```python
from build123d import *

# Parameters (mm, degrees)
SKETCH1_W                    = 57.15
SKETCH1_H                    = 38.1
BASE_FLANGE1_DEPTH           = 1.5875
EDGE_FLANGE1_STRIP_W         = 7.9375
EDGE_FLANGE1_STRIP_H         = 1.5875
EDGE_FLANGE1_STRIP_CUT_DEPTH = 57.15
EDGE_FLANGE1_DEPTH           = 57.15
F_1_4_CLEARANCE_HOLE1_D      = 6.7564
F_1_4_CLEARANCE_HOLE2_D      = 6.7564
BOSS_EXTRUDE1_DEPTH          = 57.15
CUT_EXTRUDE1_DEPTH           = 79.545162168
BOSS_EXTRUDE2_DEPTH          = 3.175
BOSS_EXTRUDE3_DEPTH          = 3.175


# Sheet-metal steps are written as plain solids
with BuildPart() as part:
    # Sketch1 → Base-Flange1 (new body)
    with BuildSketch(Plane(origin=(0, 0, 0), x_dir=(1, 0, 0), z_dir=(0, 1, 0))):
        with Locations((0, -19.05)):
            Rectangle(SKETCH1_W, SKETCH1_H)
    extrude(amount=BASE_FLANGE1_DEPTH)

    # Edge-Flange1 strip (across the edge) → Edge-Flange1 strip cut (cut)
    with BuildSketch(Plane(origin=(28.575, 1.5875, 0), x_dir=(0, 0, 1), z_dir=(-1, 0, 0))):
        with Locations((-1.5875, -0.79375)):
            Rectangle(EDGE_FLANGE1_STRIP_W, EDGE_FLANGE1_STRIP_H)
    extrude(amount=EDGE_FLANGE1_STRIP_CUT_DEPTH, mode=Mode.SUBTRACT)

    # Edge-Flange1 section (across the edge) → Edge-Flange1 (add)
    with BuildSketch(Plane(origin=(28.575, 1.5875, 0), x_dir=(0, 0, 1), z_dir=(-1, 0, 0))):
        with BuildLine():
            Line((0, 0.79375), (0, 36.5125))
            Line((0, 36.5125), (1.5875, 36.5125))
            Line((1.5875, 36.5125), (1.5875, 0.79375))
            ThreePointArc((1.5875, 0.79375), (1.819983992, 0.232483992), (2.38125, 0))
            Line((2.38125, 0), (2.38125, -1.5875))
            ThreePointArc((2.38125, -1.5875), (0.697451977, -0.890048023), (0, 0.79375))
        make_face()
    extrude(amount=EDGE_FLANGE1_DEPTH)

    # 1/4 Clearance Hole1 (through all)
    with Locations(Plane(origin=(0, 1.5875, 0), x_dir=(1, 0, 0), z_dir=(0, 1, 0))):
        with Locations((-15.875, -25.4), (15.875, -25.4)):
            Hole(F_1_4_CLEARANCE_HOLE1_D / 2)

    # 1/4 Clearance Hole2 (through all)
    with Locations(Plane.XY.offset(1.5875)):
        with Locations((-15.875, 25.4), (15.875, 25.4)):
            Hole(F_1_4_CLEARANCE_HOLE2_D / 2)

    # Sketch16 → Boss-Extrude1 (add, through all)
    with BuildSketch(Plane(origin=(28.575, 0, 0), x_dir=(0, 0, -1), z_dir=(1, 0, 0))):
        with BuildLine():
            Line((0, 2.38125), (0, 0))
            Line((0, 0), (-2.38125, 0))
            ThreePointArc((-2.38125, 0), (-0.697451977, 0.697451977), (0, 2.38125))
        make_face()
    extrude(amount=-BOSS_EXTRUDE1_DEPTH)

    # Sketch18 → Cut-Extrude1 (cut, through all)
    with BuildSketch(Plane(origin=(28.575, 0, 0), x_dir=(0, 0, -1), z_dir=(1, 0, 0))):
        with BuildLine():
            Line((-2.38125, 1.5875), (-1.5875, 1.5875))
            Line((-1.5875, 1.5875), (-1.5875, 2.38125))
            ThreePointArc((-1.5875, 2.38125), (-1.819983992, 1.819983992), (-2.38125, 1.5875))
        make_face()
    extrude(amount=-CUT_EXTRUDE1_DEPTH, mode=Mode.SUBTRACT)

    # Sketch21 → Boss-Extrude2 (add)
    with BuildSketch(Plane(origin=(28.575, 0, 0), x_dir=(0, 0, -1), z_dir=(1, 0, 0))):
        Polygon((-1.5875, 1.5875), (-38.1, 1.5875), (-38.1, 0), (0, 0), (0, 38.1), (-1.5875, 38.1), align=None)
    extrude(amount=-BOSS_EXTRUDE2_DEPTH)

    # Sketch22 → Boss-Extrude3 (add)
    with BuildSketch(Plane.ZY.offset(28.575)):
        Polygon((38.1, 1.5875), (1.5875, 1.5875), (1.5875, 38.1), (0, 38.1), (0, 0), (38.1, 0), align=None)
    extrude(amount=-BOSS_EXTRUDE3_DEPTH)


solid = part.part
```
The model under review builds one solid part; all positions refer to its coordinate system, in mm. A direction names the side the tool comes from. Give positions to 0.01 mm unless a question says otherwise; leave off trailing zeros. Write each loop counter-clockwise with the first axis right and the second up, starting at its lowest first coordinate (ties: lowest second). Pieces come first, ordered by that corner, then holes. Notation, with made-up numbers: (84, 62) - (127, 62) arc R17 ccw to (127, 92) - close; hole circle Ø8 at (89.25, 87.5). An arc over 180 degrees is marked (long way). Answer in a Markdown table with one row per item. Add a question column.
1. Tool access review of faces 5 (the flat face through (0, 1.588, 20)), 6 (the flat face through (0, 1, 38.1)): name each direction out of +Z, -Z, +X, -X, +Y, -Y from which nothing blocks a thin tool from reaching the whole face with its end or side.
2. We need section C-C on x = 16.5. Write out the cut boundary in (y, z), then the cut area to 3 significant figures.
3. We need section A-A on z = 25.4. Write out the cut boundary in (x, y) (1 decimal), then the cut area to 3 significant figures.
4. We need section D-D on z = 34. Write out the cut boundary in (x, y) (1 decimal).
5. Insertion check: P1, Ø6, axis at x = -6, z = 32, coming from the +Y side; P2, Ø5.5, axis at x = -15.875, y = 25.4, coming from the +Z side; P3, Ø11, axis at x = 14, y = 11, coming from the +Z side. Each pin has a flat end and moves straight along its axis. Give the tip position at first contact, or say it passes through.
6. Wall thickness on line 1 along Z through (x, y) = (-3.5, 8): over which ranges is the line inside the solid? List them lowest first. Write a range as [from, to].
7. Draft analysis for pull direction Z (two halves, no side actions). For faces 1 (the flat face through (0, 19, 0)), 2 (the flat face through (-28.575, 11, 1)), 3 (the cylindrical face through (-17.43, 0.78, 28.4)), 4 (the cylindrical face through (14.32, 0.78, 28.4)), state which applies: +Z half, -Z half, draft (parallel to the pull), parting line (faces both ways), or undercut.
Ans:
| question | item | result |
|---|---|---|
| 1 | face 5 | +Z, +X, -X, +Y |
| 1 | face 6 | +Z, +X, -X, +Y, -Y |
| 2 | outline | (0, 0) - (22.08, 0) - (22.08, 1.59) - (1.59, 1.59) - (1.59, 22.08) - (0, 22.08) - close; (0, 28.72) - (1.59, 28.72) - (1.59, 38.1) - (0, 38.1) - close; (28.72, 0) - (38.1, 0) - (38.1, 1.59) - (28.72, 1.59) - close |
| 2 | area | 97.4 mm^2 |
| 3 | outline | (-28.6, 0) - (-19.3, 0) - (-19.3, 1.6) - (-28.6, 1.6) - close; (-12.5, 0) - (12.5, 0) - (12.5, 1.6) - (-12.5, 1.6) - close; (19.3, 0) - (28.6, 0) - (28.6, 1.6) - (19.3, 1.6) - close |
| 3 | area | 69.3 mm^2 |
| 4 | outline | (-28.6, 0) - (28.6, 0) - (28.6, 1.6) - (-28.6, 1.6) - close |
| 5 | P1 | stops at y = 1.59 |
| 5 | P2 | passes through |
| 5 | P3 | stops at z = 1.59 |
| 6 | line 1 | z = [0, 1.59] |
| 7 | face 1 | -Z half |
| 7 | face 2 | draft |
| 7 | face 3 | undercut |
| 7 | face 4 | undercut |
